Geometry: final body of the model. Coordinates: model frame, mm. A direction names the side the tool comes from. Give positions to 0.01 mm unless a question says otherwise; leave off trailing zeros. Loops run counter-clockwise (first coordinate to the right, second up) from the corner with the lowest first, then second, coordinate; pieces in that order, holes last.
1. Section B-B, the plane y = 55. Output: boundary loops of the cut face in (x, z), then the cut area to 3 significant figures.
2. Material intervals for line 1 along Y through (x, z) = (18.5, 14.75); line 2 along X through (y, z) = (36, 7.25), sorted ascending.
3. Access query for faces 1 (the face through (7, 15, 5)), 2 (the face through (5, 30, 15)), 3 (the face through (15, 20, 15)). Directions: +Z, -Z, +X, -X, +Y, -Y. A direction counts if a zero-diameter tool reaches every point of the face in a straight line with its end or side. Return the directions, or none.
4. First-contact query: P1, Ø6, axis at y = 15, z = 12.5, coming from the +X side; P2, Ø12, axis at x = 11, y = 13, coming from the -Z side; P3, Ø2.5, axis at x = 17.5, z = 7.5, coming from the -Y side. Flat tips, straight axial feed; report the tip coordinate or a pass-through.
5. Section A-A, the plane z = 18. Output: boundary loops of the cut face in (x, y).
Autodesk Inventor part; units mm, degrees
ref_plane "YZ Plane" through (0, 0, 0) normal (1, 0, 0) x (0, 1, 0)
ref_plane "XZ Plane" through (0, 0, 0) normal (0, 1, 0) x (-1, 0, 0)
ref_plane "XY Plane" through (0, 0, 0) normal (0, 0, 1) x (1, 0, 0)
sketch "Náčrt1" plane through (0, 0, 0) normal (0, 0, 1) x (1, 0, 0)
  line L0 (0, 0) -> (20, 0)
  line L1 (20, 0) -> (20, 60)
  line L2 (20, 60) -> (0, 60)
  line L3 (0, 60) -> (0, 0)
  dimension "d0" = 20
  dimension "d1" = 60
extrude "Vysunutí1" add sketch "Náčrt1" along normal blind 25
sketch "Náčrt2" plane through (0, 0, 25) normal (0, 0, 1) x (1, 0, 0)
  line L0 (20, 60) -> (0, 60)
  line L1 (0, 0) -> (20, 0)
  line L2 (0, 60) -> (10, 60)
  line L3 (10, 60) -> (10, 0)
  line L4 (10, 0) -> (0, 0)
  line L5 (0, 0) -> (0, 60)
  dimension "d4" = 10
extrude "Vysunutí2" cut sketch "Náčrt2" against normal blind 10
sketch "Náčrt3" plane through (0, 0, 0) normal (-1, 0, 0) x (0, 0, 1)
  line L0 (0, 0) -> (25, 0)
  line L1 (0, 0) -> (5, 0)
  line L2 (5, 0) -> (5, 30)
  line L3 (5, 30) -> (0, 30)
  line L4 (0, 30) -> (0, 0)
  dimension "d7" = 5
  dimension "d8" = 30
extrude "Vysunutí3" cut sketch "Náčrt3" against normal through all
sketch "Náčrt4" plane through (0, 0, 25) normal (0, 0, 1) x (1, 0, 0)
  line L0 (20, 0) -> (20, 60)
  line L1 (20, 0) -> (15, 0)
  line L2 (15, 0) -> (15, 40)
  line L3 (15, 40) -> (20, 40)
  line L4 (20, 40) -> (20, 0)
  point P0 (0, 0)
  dimension "d11" = 5
  dimension "d12" = 40
extrude "Vysunutí4" cut sketch "Náčrt4" against normal through all
properties part number "Součást3"
Answers below:
1. outline: (0, 0) - (20, 0) - (20, 25) - (10, 25) - (10, 15) - (0, 15) - close
1. area: 400 mm2
2. line 1: y = 40 to 60
2. line 2: x = 0 to 15
3. face 1: -Z, +X, -X, -Y
3. face 2: +Z, -X, +Y, -Y
3. face 3: +Z, -Z, +X, -Y
4. P1: stops at x = 15
4. P2: stops at z = 5
4. P3: stops at y = 40
5. outline: (10, 0) - (15, 0) - (15, 40) - (20, 40) - (20, 60) - (10, 60) - close
